Verification items for the finished model (mm, model axes). Face numbers are marked on the shaded views. A direction names the side the tool comes from. Give positions to 0.01 mm unless a question says otherwise; leave off trailing zeros. Order: outer loops, then holes, each group sorted by start corner. A loop starts at its lowest first (then second) coordinate and runs counter-clockwise, first axis right, second up. Notation, with made-up numbers: (71.25, 14.25) -> (88.25, 14.25) arc R5 cw to (88.25, 23.25) -> close; hole circle Ø3 at (-29.5, 72.25). An arc over 180 degrees is marked (long way). Return JSON: item names as keys, results as strings. Group by question number.
(1) Release check for a two-part mould opening along Z. For the marked faces 5, 6 and 7 record: pulls with the +Z half, pulls with the -Z half, needs draft (parallel to the pull), parting line crosses it, or undercut.
(2) Depth check by flat-ended pin: pin 1 Ø1.8 at (x, y) = (1, 3) entering from -Z (3 decimals); pin 2 Ø1.5 at (x, y) = (6.5, 0) entering from +Z; pin 3 Ø4 at (x, y) = (7.5, 4) entering from -Z; pin 4 Ø10 at (x, z) = (-2, 1.5) entering from +Y. Enter the tip coordinate at first touch or a pass-through.
(3) Cross-section at A-A on y = 3.5. Enter the section's corners in (x, z) (3 decimals).
(4) Thickness scan on line 1 along Z through (x, y) = (-1.5, 5.25) (3 decimals); line 2 along Y through (x, z) = (-6.75, 5.25) (3 decimals); line 3 along X through (y, z) = (-2.25, -3). Record the ranges inside material, lowest first.
(5) Cross-section at B-B on x = 0. Enter the section's corners in (y, z) (3 decimals).
(6) Tool access check on the marked faces 1, 2, 3 and 4. Record the directions out of +Z, -Z, +X, -X, +Y, -Y that give a thin tool (end or side, any length) a straight path to the whole face; none if there is none.
from build123d import *

# Parameters (mm, degrees)
SKETCH1_W           = 6.604
SKETCH1_H           = 6.604
BOSS_EXTRUDE1_DEPTH = 6.35
SKETCH2_R           = 9.525
SKETCH2_W           = 6.604
SKETCH2_H           = 6.604
BOSS_EXTRUDE2_DEPTH = 3.175
FILLET1_R           = 0.508


with BuildPart() as part:
    # Sketch1 → Boss-Extrude1 (new body)
    with BuildSketch(Plane(origin=(0, 0, 0), x_dir=(1, 0, 0), z_dir=(0, 1, 0))):
        Polygon((8.065583261, 0), (4.03279163, 6.985), (-4.03279163, 6.985), (-8.065583261, 0), (-4.03279163, -6.985), (4.03279163, -6.985), align=None)
        Rectangle(SKETCH1_W, SKETCH1_H, mode=Mode.SUBTRACT)
    extrude(amount=BOSS_EXTRUDE1_DEPTH)

    # Sketch2 → Boss-Extrude2 (add)
    with BuildSketch(Plane.XZ):
        with Locations(Location((0, 0, 0), (0, 0, 270))):
            Circle(SKETCH2_R)
        Rectangle(SKETCH2_W, SKETCH2_H, mode=Mode.SUBTRACT)
    extrude(amount=BOSS_EXTRUDE2_DEPTH)

    # Fillet1
    fillet1_edges = [part.edges().sort_by_distance(p)[0] for p in [
        (0, 6.35, -6.985),
        (-6.049187445, 6.35, -3.4925),
        (-6.049187445, 6.35, 3.4925),
        (3.302, 6.35, 0),
        (0, 6.35, -3.302),
        (-3.302, 6.35, 0),
        (0, 6.35, 3.302),
        (0, 6.35, 6.985),
        (0, -3.175, 9.525),
        (0, 0, 9.525),
        (3.302, -3.175, 0),
        (0, -3.175, 3.302),
        (-3.302, -3.175, 0),
        (0, -3.175, -3.302),
        (6.049187445, 6.35, 3.4925),
        (6.049187445, 6.35, -3.4925),
    ]]
    fillet(fillet1_edges, radius=FILLET1_R)


solid = part.part
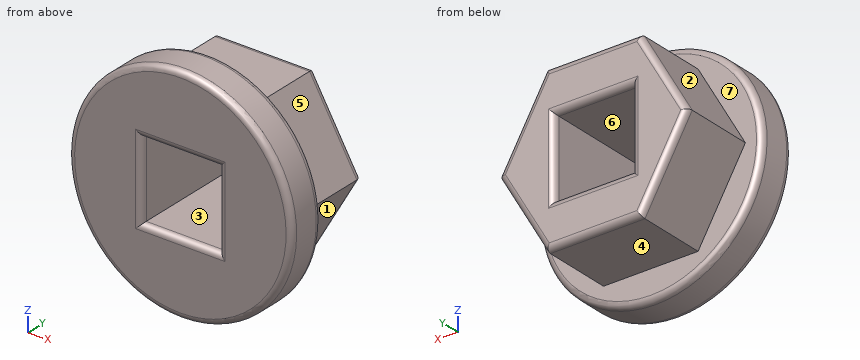
Verdict:
{
 "1": {"face 5": "pulls with the +Z half", "face 6": "undercut", "face 7": "needs draft"},
 "2": {"pin 1": "z = -6.985", "pin 2": "z = 7.5", "pin 3": "z = -4.44", "pin 4": "y = 6.35"},
 "3": {"outline": "(-8.066, 0) -> (-4.033, -6.985) -> (4.033, -6.985) -> (8.066, 0) -> (4.033, 6.985) -> (-4.033, 6.985) -> close; hole (-3.302, -3.302) -> (3.302, -3.302) -> (3.302, 3.302) -> (-3.302, 3.302) -> close"},
 "4": {"line 1": "-6.985 to -3.302, 3.302 to 6.985", "line 2": "-3.175 to 0", "line 3": "-9.04 to -3.3, 3.3 to 9.04"},
 "5": {"outline": "(-3.175, -9.017) arc R0.508 ccw to (-2.667, -9.525) -> (-0.508, -9.525) arc R0.508 ccw to (0, -9.017) -> (0, -6.985) -> (5.842, -6.985) arc R0.508 ccw to (6.35, -6.477) -> (6.35, -3.81) arc R0.508 ccw to (5.842, -3.302) -> (-2.667, -3.302) arc R0.508 ccw to (-3.175, -3.81) -> close; (-3.175, 3.81) arc R0.508 ccw to (-2.667, 3.302) -> (5.842, 3.302) arc R0.508 ccw to (6.35, 3.81) -> (6.35, 6.477) arc R0.508 ccw to (5.842, 6.985) -> (0, 6.985) -> (0, 9.017) arc R0.508 ccw to (-0.508, 9.525) -> (-2.667, 9.525) arc R0.508 ccw to (-3.175, 9.017) -> close"},
 "6": {"face 1": "-Z, +X, +Y", "face 2": "+Z, -X, +Y", "face 3": "+Y, -Y", "face 4": "-Z, +X, -X, +Y"}
}
